Read the model definition and answer for the solid it produces. Units are mm, in the model's axes. Coordinates: 2 decimals unless noted, no trailing zeros. Order: outer loops, then holes, each group sorted by start corner. A loop starts at its lowest first (then second) coordinate and runs counter-clockwise, first axis right, second up. Notation, with made-up numbers: (60.5, 57) -> (108.5, 57) arc R22 ccw to (108.5, 94) -> close; hole circle Ø10 at (69, -17.75). An arc over 180 degrees is marked (long way). Return JSON: item names as keys, results as strings. Group by question number.
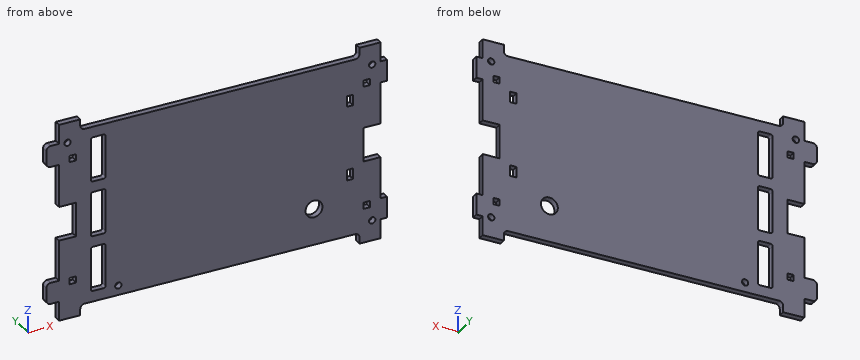
Autodesk Inventor part; units mm, degrees
ref_plane "YZ Plane" through (0, 0, 0) normal (1, 0, 0) x (0, 1, 0)
ref_plane "XZ Plane" through (0, 0, 0) normal (0, 1, 0) x (-1, 0, 0)
ref_plane "XY Plane" through (0, 0, 0) normal (0, 0, 1) x (1, 0, 0)
sketch "Sketch1" plane through (0, 0, 0) normal (0, 1, 0) x (-1, 0, 0)
  line L0 (-77, 37.5) -> (-80, 37.5)
  line L1 (-80, 27.5) -> (-77, 27.5)
  line L2 (-77, 27.5) -> (-77, 8)
  line L3 (-77, 8) -> (-69, 8)
  line L4 (-77, -37.5) -> (-80, -37.5)
  line L5 (-80, -27.5) -> (-77, -27.5)
  line L6 (-77, -27.5) -> (-77, -8)
  line L7 (-77, -8) -> (-69, -8)
  line L8 (-69, -8) -> (-69, 8)
  line L9 (-80, 37.5) -> (-80, 27.5)
  line L10 (-80, -37.5) -> (-80, -27.5)
  line L11 (75, 37.5) -> (79, 37.5)
  line L12 (81, 35.5) -> (81, 29.5)
  line L13 (79, 27.5) -> (75, 27.5)
  line L14 (75, -37.5) -> (79, -37.5)
  line L15 (81, -35.5) -> (81, -29.5)
  line L16 (79, -27.5) -> (75, -27.5)
  line L17 (75, 46.5) -> (75, 37.5)
  line L18 (75, -37.5) -> (75, -46.5)
  line L19 (-77, 37.5) -> (-77, 46.5)
  line L20 (-77, -46.5) -> (-77, -37.5)
  arc A0 (81, 35.5) -> (79, 37.5) centre (79, 35.5) ccw
  arc A1 (79, 27.5) -> (81, 29.5) centre (79, 29.5) ccw
  arc A2 (81, -29.5) -> (79, -27.5) centre (79, -29.5) ccw
  arc A3 (79, -37.5) -> (81, -35.5) centre (79, -35.5) ccw
  line L21 (75, 7.5) -> (67, 7.5)
  line L22 (67, 7.5) -> (67, -8.5)
  line L23 (67, -8.5) -> (75, -8.5)
  line L24 (75, 27.5) -> (75, 7.5)
  line L25 (75, -8.5) -> (75, -27.5)
  line L26 (-67, 46.5) -> (-67, 43.5)
  line L27 (-65, 41.5) -> (63, 41.5)
  line L28 (65, 43.5) -> (65, 46.5)
  line L29 (-77, 46.5) -> (-67, 46.5)
  line L30 (65, 46.5) -> (75, 46.5)
  line L31 (-67, -46.5) -> (-67, -43.5)
  line L32 (-65, -41.5) -> (63, -41.5)
  line L33 (65, -43.5) -> (65, -46.5)
  line L34 (-77, -46.5) -> (-67, -46.5)
  line L35 (65, -46.5) -> (75, -46.5)
  arc A4 (65, -43.5) -> (63, -41.5) centre (63, -43.5) ccw
  arc A5 (-65, -41.5) -> (-67, -43.5) centre (-65, -43.5) ccw
  arc A6 (-67, 43.5) -> (-65, 41.5) centre (-65, 43.5) ccw
  arc A7 (63, 41.5) -> (65, 43.5) centre (63, 43.5) ccw
  point P0 (0, 0)
  point P1 (81, 37.5)
  point P2 (81, 27.5)
  point P3 (81, -37.5)
  point P4 (81, -27.5)
  point P5 (-67, 41.5)
  point P6 (-67, -41.5)
  dimension "d5" = 10
  dimension "d20" = 3
  dimension "d43" = 3
  dimension "d44" = 8
  dimension "d49" = 10
  dimension "d50" = 10
  dimension "d53" = 6
  dimension "d54" = 6
  dimension "d74" = 2
  dimension "d75" = 8
  dimension "d76" = 8
  dimension "d77" = 16
  dimension "d89" = 8
  dimension "d113" = 5
  dimension "d114" = 10
  dimension "d115" = 10
  dimension "d116" = 5
  dimension "d117" = 10
  dimension "d118" = 10
  dimension "d119" = 2
  dimension "d120" = 6
  dimension "d124" = 41.5
  dimension "d127" = 6
  dimension "d128" = 80
  dimension "d129" = 3
  dimension "d130" = 132
  dimension "d133" = 3
  dimension "d135" = 33
  dimension "d136" = 93
  dimension "d140" = 16
  dimension "d142" = 8
  dimension "d144" = 10
  dimension "d145" = 5
  dimension "d146" = 5
  dimension "d147" = 27.5
  dimension "d148" = 27.5
  dimension "d149" = 27.5
  dimension "d150" = 27.5
  dimension "d164" = 161
extrude "Extrusion1" add sketch "Sketch1" along normal blind 3
sketch "Sketch2" plane through (0, 0, 0) normal (0, -1, 0) x (1, 0, 0)
  line L0 (77, 46.5) -> (77, 37.5)
  line L1 (-75, 7.5) -> (-75, 27.5)
  line L2 (-75, -27.5) -> (-75, -8.5)
  line L3 (-70, 30.5) -> (-67, 30.5)
  line L4 (-67, 30.5) -> (-67, 27.5)
  line L5 (-67, 27.5) -> (-70, 27.5)
  line L6 (-70, 27.5) -> (-70, 30.5)
  line L7 (-70, -27.5) -> (-67, -27.5)
  line L8 (-67, -27.5) -> (-67, -30.5)
  line L9 (-67, -30.5) -> (-70, -30.5)
  line L10 (-70, -30.5) -> (-70, -27.5)
  line L11 (77, -37.5) -> (77, -46.5)
  line L12 (69, 27.5) -> (72, 27.5)
  line L13 (72, 27.5) -> (72, 30.5)
  line L14 (72, 30.5) -> (69, 30.5)
  line L15 (69, 30.5) -> (69, 27.5)
  line L16 (69, -30.5) -> (72, -30.5)
  line L17 (72, -30.5) -> (72, -27.5)
  line L18 (72, -27.5) -> (69, -27.5)
  line L19 (69, -27.5) -> (69, -30.5)
  line L20 (77, -8) -> (77, -27.5)
  line L21 (77, 27.5) -> (77, 8)
  line L22 (61, 25) -> (64, 25)
  line L23 (64, 25) -> (64, 20)
  line L24 (64, 20) -> (61, 20)
  line L25 (61, 20) -> (61, 25)
  line L26 (61, -10) -> (64, -10)
  line L27 (64, -10) -> (64, -15)
  line L28 (64, -15) -> (61, -15)
  line L29 (61, -15) -> (61, -10)
  line L30 (65, -41.5) -> (-63, -41.5)
  point P0 (0, 0)
  dimension "d79" = 3
  dimension "d80" = 3
  dimension "d81" = 3
  dimension "d82" = 3
  dimension "d83" = 5
  dimension "d84" = 5
  dimension "d85" = 27.5
  dimension "d86" = 27.5
  dimension "d90" = 5
  dimension "d91" = 5
  dimension "d92" = 27.5
  dimension "d93" = 27.5
  dimension "d94" = 3
  dimension "d95" = 3
  dimension "d96" = 3
  dimension "d97" = 3
  dimension "d151" = 5
  dimension "d152" = 3
  dimension "d153" = 5
  dimension "d154" = 3
  dimension "d155" = 30
  dimension "d161" = 16
  dimension "d162" = 16
  dimension "d165" = 31.5
extrude "Extrusion5" cut sketch "Sketch2" against normal through all
sketch "Sketch4" plane through (0, 0, 0) normal (0, -1, 0) x (1, 0, 0)
  line L0 (-63, 41.5) -> (65, 41.5)
  line L1 (-75, 37.5) -> (-75, 46.5)
  line L2 (65, -41.5) -> (-63, -41.5)
  line L3 (77, -8) -> (77, -27.5)
  circle A0 centre (45.5, -24.5) radius 4
  circle A1 centre (73, 37) radius 1.5
  circle A2 centre (-71, 37) radius 1.5
  circle A3 centre (73, -37) radius 1.5
  line L4 (-75, 7.5) -> (-75, 27.5)
  line L5 (-75, -27.5) -> (-75, -8.5)
  line L6 (-59, 36.5) -> (-54, 36.5)
  line L7 (-53, 35.5) -> (-53, 16.5)
  line L8 (-54, 15.5) -> (-59, 15.5)
  line L9 (-60, 16.5) -> (-60, 35.5)
  line L10 (-59, 10.5) -> (-54, 10.5)
  line L11 (-53, 9.5) -> (-53, -9.5)
  line L12 (-54, -10.5) -> (-59, -10.5)
  line L13 (-60, -9.5) -> (-60, 9.5)
  line L14 (-59, -15.5) -> (-54, -15.5)
  line L15 (-53, -16.5) -> (-53, -35.5)
  line L16 (-54, -36.5) -> (-59, -36.5)
  line L17 (-60, -35.5) -> (-60, -16.5)
  arc A4 (-59, 36.5) -> (-60, 35.5) centre (-59, 35.5) ccw
  arc A5 (-53, 35.5) -> (-54, 36.5) centre (-54, 35.5) ccw
  arc A6 (-54, 15.5) -> (-53, 16.5) centre (-54, 16.5) ccw
  arc A7 (-60, 16.5) -> (-59, 15.5) centre (-59, 16.5) ccw
  arc A8 (-59, 10.5) -> (-60, 9.5) centre (-59, 9.5) ccw
  arc A9 (-53, 9.5) -> (-54, 10.5) centre (-54, 9.5) ccw
  arc A10 (-54, -10.5) -> (-53, -9.5) centre (-54, -9.5) ccw
  arc A11 (-60, -9.5) -> (-59, -10.5) centre (-59, -9.5) ccw
  arc A12 (-59, -15.5) -> (-60, -16.5) centre (-59, -16.5) ccw
  arc A13 (-53, -16.5) -> (-54, -15.5) centre (-54, -16.5) ccw
  arc A14 (-54, -36.5) -> (-53, -35.5) centre (-54, -35.5) ccw
  arc A15 (-60, -35.5) -> (-59, -36.5) centre (-59, -35.5) ccw
  circle A16 centre (-47, -37) radius 1.5
  point P0 (0, 0)
  point P1 (-53, 15.5)
  point P2 (-53, 36.5)
  point P3 (-60, 15.5)
  point P4 (-53, -10.5)
  point P5 (-53, 10.5)
  point P6 (-60, -10.5)
  point P7 (-53, -36.5)
  point P8 (-53, -15.5)
  point P9 (-60, -36.5)
  dimension "d167" = 17
  dimension "d168" = 8
  dimension "d169" = 3
  dimension "d170" = 3
  dimension "d171" = 144
  dimension "d172" = 4
  dimension "d173" = 31.5
  dimension "d176" = 3
  dimension "d177" = 74
  dimension "d179" = 4.5
  dimension "d181" = 4.5
  dimension "d184" = 4.5
  dimension "d185" = 21
  dimension "d186" = 7
  dimension "d187" = 15
  dimension "d188" = 5
  dimension "d189" = 21
  dimension "d190" = 7
  dimension "d191" = 5
  dimension "d192" = 15
  dimension "d193" = 21
  dimension "d194" = 5
  dimension "d195" = 15
  dimension "d196" = 7
  dimension "d197" = 1
  dimension "d200" = 3
  dimension "d201" = 4.5
  dimension "d202" = 24
extrude "Extrusion8" cut sketch "Sketch4" against normal blind 10
properties part number "Main Platform 25100813"
1. Find section B-B on z = 0. Determine the outline of the cut face in (x, y), and give its area (3 significant figures).
2. Find section D-D on y = 2.5. Give the number of separate pieces and of enclosed holes in the cut face, and give its area (3 significant figures).
3. Find section A-A on x = 45.5. Determine the outline of the cut face in (y, z).
4. Straight lines are drawn through the part: L1, parallel to Z at x = 73, y = 1.7; L2, parallel to X at y = 1.45, z = 24; L3, parallel to Z at x = 71, y = 1.05. For each, find the intervals that lie inside material, in ascending order.
5. Given pin 1 (1 mm diameter, centred on x = -38.5, y = 1.5, fed in from -Z); pin 2 (1.5 mm diameter, centred on y = 2, z = 15, fed in from -X); pin 3 (1.5 mm diameter, centred on x = 63, y = 1, fed in from +Z), each flat-ended and moving along its own axis, determine where each tip first touches the part or whether it passes through.
6. Find section C-C on z = -24.5. Determine the outline of the cut face in (x, y).
Result:
{
 "1": {"outline": "(-67, 0) -> (-60, 0) -> (-60, 3) -> (-67, 3) -> close; (-53, 0) -> (69, 0) -> (69, 3) -> (-53, 3) -> close", "area": "387 mm^2"},
 "2": {"separate pieces": "1", "enclosed holes": "14", "area": "12,200 mm^2"},
 "3": {"outline": "(0, -41.5) -> (3, -41.5) -> (3, -28.5) -> (0, -28.5) -> close; (0, -20.5) -> (3, -20.5) -> (3, 41.5) -> (0, 41.5) -> close"},
 "4": {"L1": "-46.5 to -38.5, -35.5 to -8, 8 to 35.5, 38.5 to 46.5", "L2": "-75 to -60, -53 to 61, 64 to 77", "L3": "-46.5 to -30.5, -27.5 to -8, 8 to 27.5, 30.5 to 46.5"},
 "5": {"pin 1": "z = -41.5", "pin 2": "x = -75", "pin 3": "z = 41.5"},
 "6": {"outline": "(-75, 0) -> (-60, 0) -> (-60, 3) -> (-75, 3) -> close; (-53, 0) -> (41.5, 0) -> (41.5, 3) -> (-53, 3) -> close; (49.5, 0) -> (77, 0) -> (77, 3) -> (49.5, 3) -> close"}
}
